from build123d import *

# Parameters (mm, degrees)
EXTRUDE_1_DEPTH     = 28
SKETCH_3_R          = 4.25
CUT_EXTRUDE_1_DEPTH = 61.074953184


with BuildPart() as part:
    # 草图1 → 凸台-拉伸1 (new, symmetric)
    with BuildSketch(Plane.XY):
        Polygon((0, 0), (40, 0), (40, 40), (37.5, 40), (35, 30), (35, 24.364950833), (35.6, 23.764950833), (35, 23.164950833), (35, 21.364950833), (35.6, 20.764950833), (35, 20.164950833), (35, 13), (27, 5), (19.835049167, 5), (19.235049167, 4.4), (18.635049167, 5), (16.835049167, 5), (16.235049167, 4.4), (15.635049167, 5), (10, 5), (0, 2.5), align=None)
    extrude(amount=EXTRUDE_1_DEPTH, both=True)

    # 草图3 → 切除-拉伸1 (cut, through all)
    with BuildSketch(Plane(origin=(0, 5, 0), x_dir=(1, 0, 0), z_dir=(0, 1, 0))):
        with Locations(Location((20, 15, 0), (0, 0, 270))):
            Circle(SKETCH_3_R)
        with Locations(Location((20, -15, 0), (0, 0, 267.775679771))):
            Circle(SKETCH_3_R)
    cut_extrude_1 = extrude(amount=-CUT_EXTRUDE_1_DEPTH, mode=Mode.SUBTRACT)

    # 镜向1: 切除-拉伸1 across plane
    add(cut_extrude_1.mirror(Plane(origin=(20, 20, 0), x_dir=(0, 0, 1), z_dir=(-0.7071067811865414, -0.7071067811865538, 0))), mode=Mode.SUBTRACT)


solid = part.part
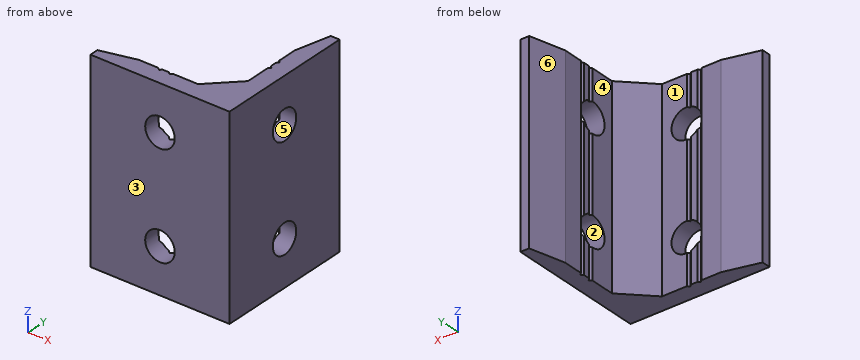
The model under review builds one solid part; all positions refer to its coordinate system, in mm. Face numbers are marked on the shaded views. A direction names the side the tool comes from. Round coordinates to 2 decimals unless told otherwise and drop trailing zeros. Write each loop counter-clockwise with the first axis right and the second up, starting at its lowest first coordinate (ties: lowest second). Pieces come first, ordered by that corner, then holes. Notation, with made-up numbers: M -26,-7.5 L 28,-7.5 A21 cw 28,0.5 Z; hole C 13.5,44 d4. An arc over 180 degrees is marked long. Use a Markdown table: item, result. Add a question column.
Q1. We need section C-C, the plane z = 8. State the section outline as (x, y) points, plus the area to 3 significant figures.
Q2. We need section B-B, the plane y = 28. State the section outline as (x, z) points, plus the area to 3 significant figures.
Q3. Insertion check: pin 1 (0.9 mm diameter, centred on y = 22.5, z = 0, fed in from -X); pin 2 (1.4 mm diameter, centred on x = 17.5, z = -3.5, fed in from +Y); pin 3 (8 mm diameter, centred on x = 28, z = 10.5, fed in from +Y). Each pin has a flat end and moves straight along its axis. Give the tip position at first contact, or say it passes through.
Q4. The part is to be moulded in two halves that separate along Y. For the marked faces 3, 4, 5 and 6, say which applies: pulls with the +Y half, pulls with the -Y half, needs draft (parallel to the pull), parting line crosses it, or undercut.
Q5. To check wall thickness, follow line 1 (Z direction, x = 20, y = 1); line 2 (Y direction, x = 38.2, z = 15); line 3 (Z direction, x = 38, y = 16.5). State the ranges of each line that lie inside material, in increasing order.
Q6. We need section D-D, the plane x = 33.5. State the section outline as (y, z) points, plus the area to 3 significant figures.
Q7. Machinability: for the marked faces 1 and 2, which of the approach directions +Z, -Z, +X, -X, +Y, -Y give a long, thin tool a straight path to every point of the face, cutting with its end or side? Answer none if there is none.
Q8. We need section A-A, the plane z = -15. State the section outline as (x, y) points, plus the area to 3 significant figures.
Findings below:
| question | item | result |
|---|---|---|
| 1 | outline | M 0,0 L 40,0 L 40,40 L 37.5,40 L 35,30 L 35,24.36 L 35.6,23.76 L 35,23.16 L 35,21.36 L 35.6,20.76 L 35,20.16 L 35,13 L 27,5 L 19.84,5 L 19.24,4.4 L 18.64,5 L 16.84,5 L 16.24,4.4 L 15.64,5 L 10,5 L 0,2.5 Z |
| 1 | area | 381 mm² |
| 2 | outline | M 35,-28 L 40,-28 L 40,28 L 35,28 Z |
| 2 | area | 280 mm² |
| 3 | pin 1 | stops at x = 35 |
| 3 | pin 2 | stops at y = 5 |
| 3 | pin 3 | stops at y = 10 |
| 4 | face 3 | pulls with the -Y half |
| 4 | face 4 | needs draft |
| 4 | face 5 | undercut |
| 4 | face 6 | pulls with the +Y half |
| 5 | line 1 | z = -28 to -19.25, -10.75 to 10.75, 19.25 to 28 |
| 5 | line 2 | y = 0 to 15.75, 24.25 to 40 |
| 5 | line 3 | z = -28 to -17.41, -12.59 to 12.59, 17.41 to 28 |
| 6 | outline | M 0,-28 L 11.5,-28 L 11.5,28 L 0,28 Z |
| 6 | area | 644 mm² |
| 7 | face 1 | +Z, -Z, -X, +Y |
| 7 | face 2 | +X, -X |
| 8 | outline | M 0,0 L 15.75,0 L 15.75,4.89 L 15.64,5 L 10,5 L 0,2.5 Z; M 24.25,0 L 40,0 L 40,15.75 L 35,15.75 L 35,13 L 27,5 L 24.25,5 Z; M 35,24.36 L 35.11,24.25 L 40,24.25 L 40,40 L 37.5,40 L 35,30 Z |
| 8 | area | 297 mm² |
